```python
from build123d import *

# Parameters (mm, degrees)
F0_W      = 209.42099
F0_H      = 52.317056
F1_DEPTH  = 150
F2_R      = 50.698485
F3_R      = 51.659231
F4_DEPTH  = 66
F5_R      = 33.468817
F6_DEPTH  = 54
F7_R      = 14.795614
F8_DEPTH  = 5
F9_R      = 10.620202
F10_DEPTH = 9
F11_W     = 34.047097
F11_H     = 17.011657
F12_DEPTH = 43
F13_W     = 25.994077
F13_H     = 15.360802
F14_DEPTH = 77


with BuildPart() as f1:
    # F0 (on Top) → F1 (new body)
    with BuildSketch(Plane.XY):
        with Locations((-55.119449, -58.706915)):
            Rectangle(F0_W, F0_H)
    extrude(amount=F1_DEPTH)

    # F2
    f2_edges = [f1.edges().sort_by_distance(p)[0] for p in [
        (49.591046, -58.706915, 150),
    ]]
    fillet(f2_edges, radius=F2_R)

    # F3 (on face) → F4 (join)
    with BuildSketch(Plane.XZ.offset(84.865443)):
        with Locations((-69.931231, 77.866942)):
            Circle(F3_R)
    extrude(amount=F4_DEPTH)

    # F5 (on face) → F6 (join)
    with BuildSketch(Plane.XZ.offset(150.865443)):
        with Locations((-69.931231, 77.866942)):
            Circle(F5_R)
    extrude(amount=F6_DEPTH)

    # F7 (on face) → F8 (join)
    with BuildSketch(Plane.XY.offset(150)):
        with Locations((-138.16677, -55.403817)):
            Circle(F7_R)
    extrude(amount=F8_DEPTH)

    # F9 (on face) → F10 (join)
    with BuildSketch(Plane.XY.offset(155)):
        with Locations((-138.16677, -55.403817)):
            Circle(F9_R)
    extrude(amount=F10_DEPTH)

    # F11 (on face) → F12 (join)
    with BuildSketch(Plane.XZ.offset(84.865443)):
        with Locations((-135.340422, 126.199729)):
            Rectangle(F11_W, F11_H)
    extrude(amount=-F12_DEPTH)

    # F13 (on face) → F14 (cut)
    with BuildSketch(Plane.XZ.offset(84.865443)):
        with Locations((-123.564697, 125.956863)):
            Rectangle(F13_W, F13_H)
    extrude(amount=-F14_DEPTH, mode=Mode.SUBTRACT)


solid = f1.part
```
Design review of the part built by this model. Coordinates are the model's own, in mm. A direction names the side the tool comes from. Give positions to 0.01 mm unless a question says otherwise; leave off trailing zeros. Write each loop counter-clockwise with the first axis right and the second up, starting at its lowest first coordinate (ties: lowest second). Pieces come first, ordered by that corner, then holes. Notation, with made-up numbers: (79.5, 48.25) - (91.5, 48.25) arc R29 ccw to (91.5, 82.25) - close; hole circle Ø10 at (-5, 33). An arc over 180 degrees is marked (long way). Return JSON: item names as keys, results as strings. Group by question number.
(1) Mouldability with a two-part tool opening along X and no side actions: class faces 1 (the flat face through (-138, -55, 164)), 2 (the flat face through (-136.562, -59, 126)), 3 (the flat face through (49.591, -59, 49)), 4 (the flat face through (-124, -59, 133.637)) as +X half, -X half, draft (parallel to the pull), parting line (faces both ways), or undercut.
(2) Machinability: for faces 5 (the flat face through (-142, -45, 155)), 6 (the cylindrical face through (-42.16, -117.403, 121.426)), 7 (the flat face through (-57, -58, 0)), 8 (the flat face through (-159.83, -59, 74)), 9 (the flat face through (-124, -59, 118.276)), which of the approach directions +Z, -Z, +X, -X, +Y, -Y give a long, thin tool a straight path to every point of the face, cutting with its end or side? Answer none if there is none.
(3) We need section A-A, the plane y = -48. Give the boundary of the cut face in (x, z), then the cut area to 3 significant figures.
(4) Insertion check: pin 1 (21 mm diameter, centred on x = -117.5, y = -69, fed in from +Z); pin 2 (12 mm diameter, centred on x = -58.5, y = -169, fed in from +Z); pin 3 (10 mm diameter, centred on x = 16.5, y = -53, fed in from +Z); pin 4 (8 mm diameter, centred on x = -124.5, y = -61, fed in from -Z). Each pin has a flat end and moves straight along its axis. Give the tip position at first contact, or say it passes through.
(5) We need section D-D, the plane x = -64.5. Give the boundary of the cut face in (y, z), then the cut area to 3 significant figures.
(6) We need section C-C, the plane z = 89.5. Give the boundary of the cut face in (x, y).
(7) To check wall thickness, follow probe 1 along Z at (x, y) = (-112.5, -47.5); probe 2 along Y at (x, z) = (-117, 112); probe 3 along X at (y, z) = (-58.5, 142). State the ranges of each line that lie inside material, in increasing order.
(8) We need section B-B, the plane x = -113.5. Give the boundary of the cut face in (y, z), then the cut area to 3 significant figures.
Reported:
{
 "1": {"face 1": "draft", "face 2": "undercut", "face 3": "+X half", "face 4": "undercut"},
 "2": {"face 5": "+Z", "face 6": "-Y", "face 7": "-Z, +X, -X, +Y, -Y", "face 8": "+Z, -Z, -X, +Y, -Y", "face 9": "+Y, -Y"},
 "3": {"outline": "(-159.83, 0) - (49.59, 0) - (49.59, 99.3) arc R50.7 ccw to (-1.11, 150) - (-125.36, 150) - (-125.36, 155) - (-130.55, 155) - (-130.55, 164) - (-145.78, 164) - (-145.78, 155) - (-150.98, 155) - (-150.98, 150) - (-159.83, 150) - close; hole (-136.56, 118.28) - (-110.57, 118.28) - (-110.57, 133.64) - (-136.56, 133.64) - close", "area": "30,700 mm2"},
 "4": {"pin 1": "stops at z = 155", "pin 2": "stops at z = 110.89", "pin 3": "stops at z = 148.41", "pin 4": "stops at z = 0"},
 "5": {"outline": "(-204.87, 44.84) - (-150.87, 44.84) - (-150.87, 26.49) - (-84.87, 26.49) - (-84.87, 0) - (-32.55, 0) - (-32.55, 150) - (-84.87, 150) - (-84.87, 129.24) - (-150.87, 129.24) - (-150.87, 110.89) - (-204.87, 110.89) - close", "area": "18,200 mm2"},
 "6": {"outline": "(-159.83, -84.87) - (-120.26, -84.87) - (-120.26, -150.87) - (-101.31, -150.87) - (-101.31, -204.87) - (-38.55, -204.87) - (-38.55, -150.87) - (-19.6, -150.87) - (-19.6, -84.87) - (49.59, -84.87) - (49.59, -32.55) - (-159.83, -32.55) - close"},
 "7": {"probe 1": "z = 0 to 118.28, 133.64 to 150", "probe 2": "y = -84.87 to -32.55", "probe 3": "x = -159.83 to 26.23"},
 "8": {"outline": "(-150.87, 50.11) - (-84.87, 50.11) - (-84.87, 0) - (-32.55, 0) - (-32.55, 118.28) - (-84.87, 118.28) - (-84.87, 105.62) - (-150.87, 105.62) - close; (-84.87, 133.64) - (-32.55, 133.64) - (-32.55, 150) - (-84.87, 150) - close", "area": "10,700 mm2"}
}
